Read the model definition and answer for the solid it produces. Units are mm, in the model's axes. Give positions to 0.01 mm unless a question says otherwise; leave off trailing zeros. Order: outer loops, then holes, each group sorted by start corner. A loop starts at its lowest first (then second) coordinate and runs counter-clockwise, first axis right, second up. Notation, with made-up numbers: (71, -14) - (106, -14) arc R22 ccw to (106, 12) - close; hole circle Ø2 at (76, -37). An arc over 180 degrees is marked (long way). Return JSON: item names as keys, results as strings.
Autodesk Inventor part; units mm, degrees
ref_plane "YZ Plane" through (0, 0, 0) normal (1, 0, 0) x (0, 1, 0)
ref_plane "XZ Plane" through (0, 0, 0) normal (0, 1, 0) x (-1, 0, 0)
ref_plane "XY Plane" through (0, 0, 0) normal (0, 0, 1) x (1, 0, 0)
sketch "Sketch1" plane through (0, 0, 0) normal (0, 1, 0) x (-1, 0, 0)
  line L0 (0, 50) -> (0, -50) construction
  line L1 (-5, 50) -> (-5, -50)
  line L2 (5, -50) -> (5, 50)
  arc A0 (5, 50) -> (-5, 50) centre (0, 50) ccw
  arc A1 (-5, -50) -> (5, -50) centre (0, -50) ccw
  circle A2 centre (0, 50) radius 2.5
  circle A3 centre (0, 0) radius 2.5
  circle A4 centre (0, -50) radius 2.5
  dimension "d0" = 50
  dimension "d1" = 10
  dimension "d2" = 5
  dimension "d3" = 5
  dimension "d4" = 5
extrude "Extrusion1" add sketch "Sketch1" along normal blind 3
properties part number "Lazy Tongs beam Long"
Q1. A cutting plane is placed at B-B (x = 0). Write down the section's boundary in (y, z).
Values:
{"outline": "(0, -55) - (3, -55) - (3, -52.5) - (0, -52.5) - close; (0, -47.5) - (3, -47.5) - (3, -2.5) - (0, -2.5) - close; (0, 2.5) - (3, 2.5) - (3, 47.5) - (0, 47.5) - close; (0, 52.5) - (3, 52.5) - (3, 55) - (0, 55) - close"}
Q2. A cutting plane is placed at C-C (z = 0). Write down the section's boundary in (x, y).
Values:
{"outline": "(-5, 0) - (-2.5, 0) - (-2.5, 3) - (-5, 3) - close; (2.5, 0) - (5, 0) - (5, 3) - (2.5, 3) - close"}
Q3. Given pin 1 (1 mm diameter, centred on x = 0.5, y = 2.5, fed in from -Z); pin 2 (4.5 mm diameter, centred on x = 0, z = 50, fed in from -Y), each flat-ended and moving along its own axis, determine where each tip first touches the part or whether it passes through.
Values:
{"pin 1": "stops at z = -55", "pin 2": "passes through"}
Q4. A cutting plane is placed at A-A (y = 1.7). Write down the section's boundary in (x, z).
Values:
{"outline": "(-5, -50) arc R5 ccw to (5, -50) - (5, 50) arc R5 ccw to (-5, 50) - close; hole circle Ø5 at (0, -50); hole circle Ø5 at (0, 0); hole circle Ø5 at (0, 50)"}
Q5. Consider L1, parallel to Z at x = 0.25, y = 2.2; L2, parallel to Z at x = 1.75, y = 1; L3, parallel to X at y = 0.4, z = 2. Determine where each line is inside the solid, lowest interval first.
Values:
{"L1": "z = -54.99 to -52.49, -47.51 to -2.49, 2.49 to 47.51, 52.49 to 54.99", "L2": "z = -54.68 to -51.79, -48.21 to -1.79, 1.79 to 48.21, 51.79 to 54.68", "L3": "x = -5 to -1.5, 1.5 to 5"}
Q6. Determine the mould class of faces 1 (the cylindrical face through (0.54, 1.48, 2.44)), 2 (the cylindrical face through (0, 1, 55)), 3 (the flat face through (5, 1, 1)) for opening direction Z: released by +Z, released by -Z, zero draft, split by the parting line, or undercut.
Values:
{"face 1": "undercut", "face 2": "released by +Z", "face 3": "zero draft"}
